Job drawing, mm, ordinate dimensions from the low corner. One solid piece. A direction names the side the tool comes from. Coordinates: 2 decimals unless noted, no trailing zeros. Write each loop counter-clockwise with the first axis right and the second up, starting at its lowest first coordinate (ties: lowest second). Pieces come first, ordered by that corner, then holes. Notation, with made-up numbers: (79.5, 10.25) - (84.5, 10.25) arc R22 ccw to (84.5, 35.25) - close; hole circle Ø6 at (10.25, 44). An arc over 180 degrees is marked (long way). Use one line per item in the form item = value. Start each with the question number.
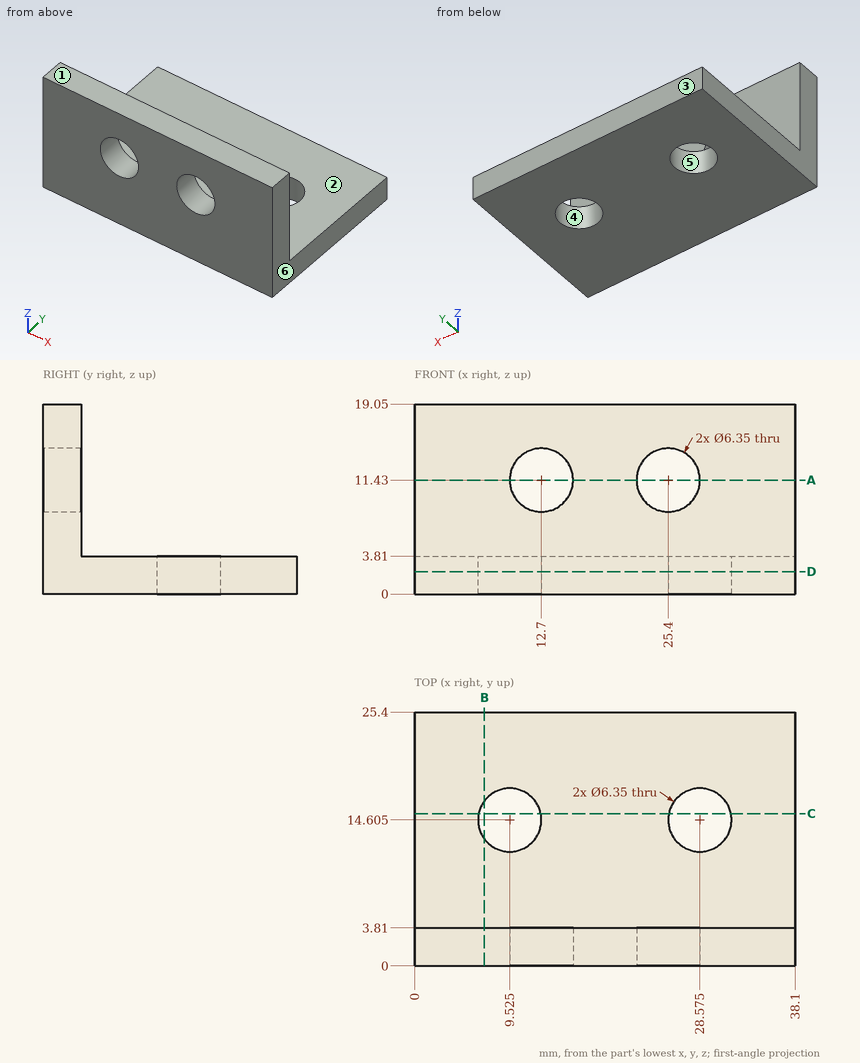
Q1. Pin check, flat tips, straight feed: P1, Ø5, axis at x = 31.5, z = 12.5, coming from the -Y side; P2, Ø7.5, axis at x = 25.4, z = 11.43, coming from the +Y side; P3, Ø11, axis at x = 26.5, y = 12.5, coming from the +Z side. Stop position of each tip, or through.
Q2. Which spindle directions (+Z, -Z, +X, -X, +Y, -Y) get a long thin tool onto all of the face, cutting with end or side? Do the marked faces 1 and 2. Say none if no direction does.
Q3. Drill centre lines: probe 1 along X at (y, z) = (1.2, 11.43) (3 decimals); probe 2 along Z at (x, y) = (7.5, 7.5). Where is each one in solid material? Low to high.
Q4. Slice it at D-D (z = 2.25). List the corners of the cut face in (x, y) (3 decimals), plus the area to 3 significant figures.
Q5. Slice it at A-A (z = 11.43). List the corners of the cut face in (x, y) (3 decimals), plus the area to 3 significant figures.
Q6. Slice it at B-B (x = 7). List the corners of the cut face in (y, z).
Q7. Mould opens along Y. For the marked faces 3, 4, 5 and 6 say: released by +Y, released by -Y, zero draft, split by the parting line, or undercut.
Q8. Slice it at C-C (y = 15.25). List the corners of the cut face in (x, z).
Solution:
q1.P1 = 0
q1.P2 = 3.81
q1.P3 = 3.81
q2.face_1 = +Z, +X, -X, +Y, -Y
q2.face_2 = +Z, +X, -X, +Y
q3.probe_1 = 0 to 9.525, 15.875 to 22.225, 28.575 to 38.1
q3.probe_2 = 0 to 3.81
q4.outline = (0, 0) - (38.1, 0) - (38.1, 25.4) - (0, 25.4) - close; hole circle Ø6.35 at (9.525, 14.605); hole circle Ø6.35 at (28.575, 14.605)
q4.area = 904 mm2
q5.outline = (0, 0) - (9.525, 0) - (9.525, 3.81) - (0, 3.81) - close; (15.875, 0) - (22.225, 0) - (22.225, 3.81) - (15.875, 3.81) - close; (28.575, 0) - (38.1, 0) - (38.1, 3.81) - (28.575, 3.81) - close
q5.area = 96.8 mm2
q6.outline = (0, 0) - (12.68, 0) - (12.68, 3.81) - (3.81, 3.81) - (3.81, 19.05) - (0, 19.05) - close; (16.53, 0) - (25.4, 0) - (25.4, 3.81) - (16.53, 3.81) - close
q7.face_3 = released by +Y
q7.face_4 = undercut
q7.face_5 = undercut
q7.face_6 = zero draft
q8.outline = (0, 0) - (6.42, 0) - (6.42, 3.81) - (0, 3.81) - close; (12.63, 0) - (25.47, 0) - (25.47, 3.81) - (12.63, 3.81) - close; (31.68, 0) - (38.1, 0) - (38.1, 3.81) - (31.68, 3.81) - close
